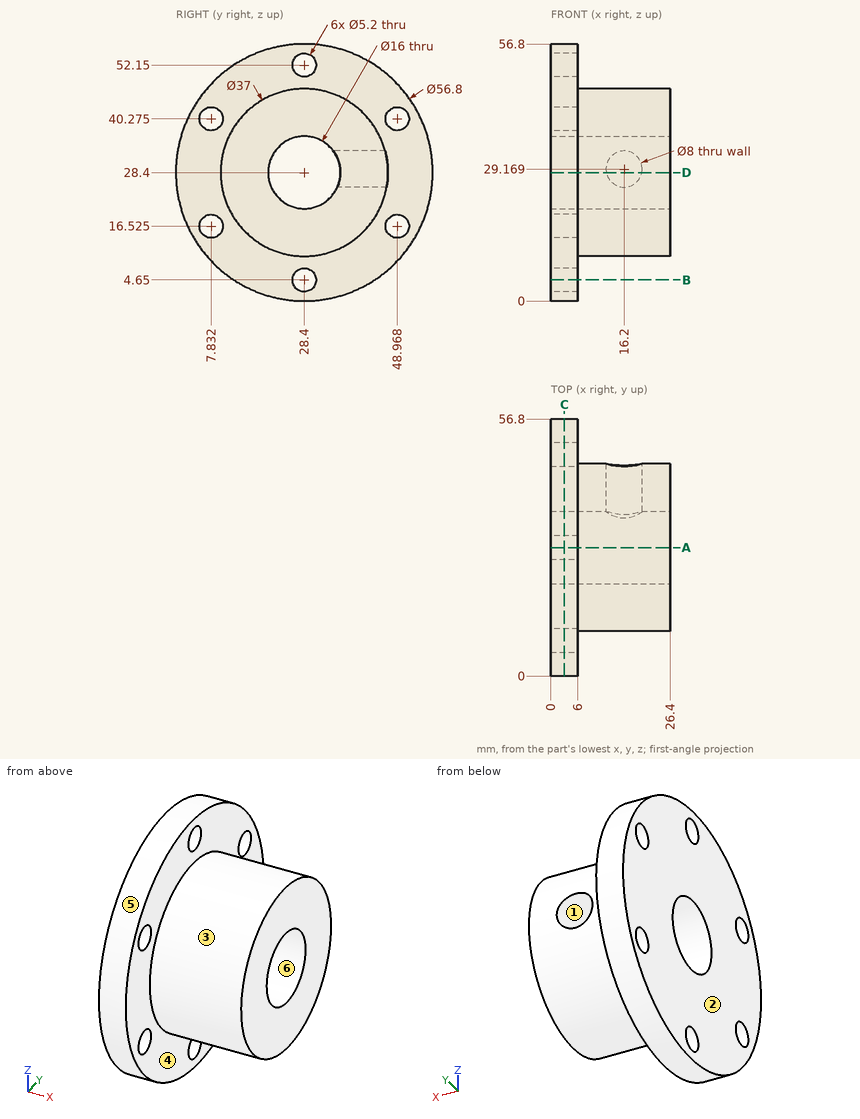
The figure shows three views and two pictorial views of one solid part (mm, origin at its lowest corner). Answer the questions. A direction names the side the tool comes from. Coordinates: 2 decimals unless noted, no trailing zeros. Loops run counter-clockwise (first coordinate to the right, second up) from the corner with the lowest first, then second, coordinate; pieces in that order, holes last. Notation, with made-up numbers: (-22.5, -5.75) -> (-11.5, -5.75) arc R33 ccw to (-11.5, 30.25) -> close; hole circle Ø8 at (-39, 15.25). An arc over 180 degrees is marked (long way). Write item = value, one per line. Start each with the question number.
1) A cutting plane is placed at B-B (z = 4.65). Give the vertices of the cut face in (x, y).
2) A cutting plane is placed at C-C (x = 3). Give the vertices of the cut face in (y, z) (3 decimals).
3) A tool of negligible diameter and unlimited length cuts with its end or side. For the marked faces 1, 2 and 3, from which of +Z, -Z, +X, -X, +Y, -Y can it reach the whole face along a straight path? Write none if from no direction.
4) Straight lines are drawn through the part: line 1 (Z direction, x = 4.5, y = 28.4); line 2 (Z direction, x = 3.75, y = 27.5); line 3 (Z direction, x = 23.25, y = 28.5). For each, find the intervals that lie inside material, in ascending order. Write a range as from..to.
5) A cutting plane is placed at A-A (y = 28.4). Give the vertices of the cut face in (x, z), then the cut area to 3 significant figures.
6) Given pin 1 Ø5 at (x, z) = (16.2, 29.17) entering from +Y; pin 2 Ø1 at (x, y) = (18.5, 14) entering from -Z; pin 3 Ø1 at (x, y) = (11, 23.5) entering from -Z; pin 4 Ø4 at (y, z) = (48.97, 40.28) entering from +X, each flat-ended and moving along its own axis, determine where each tip first touches the part or whether it passes through.
7) A cutting plane is placed at D-D (z = 28.4). Give the vertices of the cut face in (x, y) (1 decimal).
8) The mould has two halves that part along Z. Classify the marked faces 4, 5 and 6: released by +Z, released by -Z, zero draft, split by the parting line, or undercut.
Responses:
q1.outline = (0, 12.83) -> (6, 12.83) -> (6, 25.8) -> (0, 25.8) -> close; (0, 31) -> (6, 31) -> (6, 43.97) -> (0, 43.97) -> close
q2.outline = circle Ø56.8 at (28.4, 28.4); hole circle Ø5.2 at (7.832, 16.525); hole circle Ø5.2 at (7.832, 40.275); hole circle Ø16 at (28.4, 28.4); hole circle Ø5.2 at (28.4, 4.65); hole circle Ø5.2 at (28.4, 52.15); hole circle Ø5.2 at (48.968, 16.525); hole circle Ø5.2 at (48.968, 40.275)
q3.face_1 = +Y
q3.face_2 = +Z, -Z, -X, +Y, -Y
q3.face_3 = +X
q4.line_1 = 0..2.05, 7.25..20.4, 36.4..49.55, 54.75..56.8
q4.line_2 = 0.01..2.21, 7.09..20.45, 36.35..49.71, 54.59..56.79
q4.line_3 = 9.9..20.4, 36.4..46.9
q5.outline = (0, 0) -> (6, 0) -> (6, 2.05) -> (0, 2.05) -> close; (0, 7.25) -> (6, 7.25) -> (6, 9.9) -> (26.4, 9.9) -> (26.4, 20.4) -> (0, 20.4) -> close; (0, 36.4) -> (26.4, 36.4) -> (26.4, 46.9) -> (6, 46.9) -> (6, 49.55) -> (0, 49.55) -> close; (0, 54.75) -> (6, 54.75) -> (6, 56.8) -> (0, 56.8) -> close
q5.area = 611 mm²
q6.pin_1 = 21.1
q6.pin_2 = 16.19
q6.pin_3 = 10.43
q6.pin_4 = through
q7.outline = (0, 0) -> (6, 0) -> (6, 9.9) -> (26.4, 9.9) -> (26.4, 20.4) -> (0, 20.4) -> close; (0, 36.4) -> (12.3, 36.4) -> (12.3, 46.9) -> (6, 46.9) -> (6, 56.8) -> (0, 56.8) -> close; (20.1, 36.4) -> (26.4, 36.4) -> (26.4, 46.9) -> (20.1, 46.9) -> close
q8.face_4 = zero draft
q8.face_5 = split by the parting line
q8.face_6 = undercut
